Build history of the part. All positions in model axes, mm. Face numbers are marked on the shaded views. A direction names the side the tool comes from. Coordinates: 2 decimals unless noted, no trailing zeros. Order: outer loops, then holes, each group sorted by start corner. A loop starts at its lowest first (then second) coordinate and runs counter-clockwise, first axis right, second up. Notation, with made-up numbers: (6.5, 14) - (38.5, 14) arc R21 cw to (38.5, 30) - close; hole circle Ø1 at (21, 19.25). An arc over 180 degrees is marked (long way). Return JSON: item names as keys, results as strings.
from build123d import *

# Parameters (mm, degrees)
SKETCH1_W               = 12
SKETCH1_H               = 6.5
BOSS_EXTRUDE1_DEPTH     = 10
SKETCH2_W               = 16
SKETCH2_H               = 10.5
BOSS_EXTRUDE2_DEPTH     = 15
SKETCH3_W               = 9
SKETCH3_H               = 2.5
CUT_EXTRUDE1_DEPTH      = 10
CUT_EXTRUDE2_DEPTH      = 19.027756377
CUT_EXTRUDE2_DEPTH_BACK = 19.027756377
SKETCH4_W               = 5
SKETCH4_H               = 5.5


with BuildPart() as part:
    # Sketch1 → Boss-Extrude1 (new body)
    with BuildSketch(Plane(origin=(0, 0, 0), x_dir=(1, 0, 0), z_dir=(0, 1, 0))):
        Rectangle(SKETCH1_W, SKETCH1_H)
    extrude(amount=BOSS_EXTRUDE1_DEPTH)

    # Sketch2 → Boss-Extrude2 (add)
    with BuildSketch(Plane(origin=(0, 0, 0), x_dir=(1, 0, 0), z_dir=(0, 1, 0))):
        Rectangle(SKETCH2_W, SKETCH2_H)
    extrude(amount=-BOSS_EXTRUDE2_DEPTH)

    # Sketch3 → Cut-Extrude1 (cut)
    with BuildSketch(Plane(origin=(0, 10, 0), x_dir=(1, 0, 0), z_dir=(0, 1, 0))):
        with Locations((0, 2)):
            Rectangle(SKETCH3_W, SKETCH3_H)
        with Locations((0, -2)):
            Rectangle(SKETCH3_W, SKETCH3_H)
    extrude(amount=-CUT_EXTRUDE1_DEPTH, mode=Mode.SUBTRACT)

    # Sketch4 → Cut-Extrude2 (cut, two sides: drawn at the far end of the back side and taken through both)
    with BuildSketch(Plane(origin=(0, 0, -0.75), x_dir=(-1, 0, 0), z_dir=(0, 0, -1)).offset(-CUT_EXTRUDE2_DEPTH_BACK)):
        with Locations((0, 3.75)):
            Rectangle(SKETCH4_W, SKETCH4_H)
    extrude(amount=CUT_EXTRUDE2_DEPTH + CUT_EXTRUDE2_DEPTH_BACK, mode=Mode.SUBTRACT)


solid = part.part
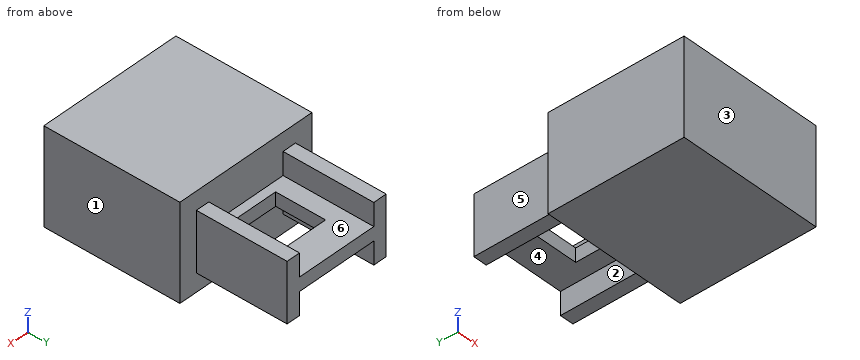
1. Cut at D-D on x = 3.25. Give the cut face in (y, z).
Check values:
{"outline": "(-15, -5.25) - (0, -5.25) - (0, -0.75) - (10, -0.75) - (10, 0.75) - (0, 0.75) - (0, 5.25) - (-15, 5.25) - close"}
2. Probe L1, parallel to X at y = 4, z = 3; L2, parallel to Y at x = -1.25, z = 0.25; L3, parallel to X at y = 6, z = 0. List the from-to ranges inside material, lowest first.
Check values:
{"L1": "-6 to -4.5, 4.5 to 6", "L2": "-15 to 1, 6.5 to 10", "L3": "-6 to -2.5, 2.5 to 6"}
3. Cut at C-C on z = -2. Give the cut face in (x, y), plus the area to 3 significant figures.
Check values:
{"outline": "(-8, -15) - (8, -15) - (8, 0) - (6, 0) - (6, 10) - (4.5, 10) - (4.5, 0) - (-4.5, 0) - (-4.5, 10) - (-6, 10) - (-6, 0) - (-8, 0) - close", "area": "270 mm²"}
4. Tool access for the marked faces 4, 5 and 6: list every direction of +Z, -Z, +X, -X, +Y, -Y with a clear straight run to the whole face (end or side of a thin tool).
Check values:
{"face 4": "-Z, +Y", "face 5": "+Z, -Z, -X, +Y", "face 6": "+Z, +Y"}
5. Cut at B-B on y = 5. Give the cut face in (x, z).
Check values:
{"outline": "(-6, -3.25) - (-4.5, -3.25) - (-4.5, -0.75) - (-2.5, -0.75) - (-2.5, 0.75) - (-4.5, 0.75) - (-4.5, 3.25) - (-6, 3.25) - close; (2.5, -0.75) - (4.5, -0.75) - (4.5, -3.25) - (6, -3.25) - (6, 3.25) - (4.5, 3.25) - (4.5, 0.75) - (2.5, 0.75) - close"}
6. Drop flat-ended pins along their axis: pin 1 (3 mm diameter, centred on y = 5, z = 2, fed in from +X); pin 2 (1.6 mm diameter, centred on x = 5.5, y = 4, fed in from +Z); pin 3 (3 mm diameter, centred on y = 6, z = 2, fed in from -X). Give the stop position or say it passes through.
Check values:
{"pin 1": "x = 6", "pin 2": "z = 3.25", "pin 3": "x = -6"}
7. Cut at A-A on x = 0. Give the cut face in (y, z), plus the area to 3 significant figures.
Check values:
{"outline": "(-15, -5.25) - (0, -5.25) - (0, -0.75) - (1, -0.75) - (1, 0.75) - (0, 0.75) - (0, 5.25) - (-15, 5.25) - close; (6.5, -0.75) - (10, -0.75) - (10, 0.75) - (6.5, 0.75) - close", "area": "164 mm²"}
8. Mould opens along X. For the marked faces 1, 2 and 3 say: pulls with the +X half, pulls with the -X half, needs draft (parallel to the pull), parting line crosses it, or undercut.
Check values:
{"face 1": "pulls with the +X half", "face 2": "undercut", "face 3": "needs draft"}
